from build123d import *

# Parameters (mm, degrees)
SKETCH1_R           = 4
SKETCH1_R_2         = 2.525
BOSS_EXTRUDE1_DEPTH = 5.1
BOSS_EXTRUDE2_DEPTH = 6.4
SKETCH3_R           = 2.5
BOSS_EXTRUDE5_DEPTH = 1.1


with BuildPart() as part:
    # Sketch1 → Boss-Extrude1 (new body)
    with BuildSketch(Plane.XY):
        Circle(SKETCH1_R)
        Circle(SKETCH1_R_2, mode=Mode.SUBTRACT)
    extrude(amount=BOSS_EXTRUDE1_DEPTH)

    # Sketch2 → Boss-Extrude2 (add)
    with BuildSketch(Plane(origin=(0, 0, 0), x_dir=(-1, 0, 0), z_dir=(0, 0, -1))):
        Polygon((-1.7, 3.4), (-1.7, 1.7), (-3.4, 1.7), (-3.4, -1.7), (-1.7, -1.7), (-1.7, -3.4), (1.7, -3.4), (1.7, -1.7), (3.4, -1.7), (3.4, 1.7), (1.7, 1.7), (1.7, 3.4), align=None)
        with BuildLine():
            Line((-1.05, 2.45), (-1.05, 1.55))
            ThreePointArc((-1.05, 1.55), (-1.196446609, 1.196446609), (-1.55, 1.05))
            Line((-1.55, 1.05), (-2.45, 1.05))
            Line((-2.45, 1.05), (-2.45, -1.05))
            Line((-2.45, -1.05), (-1.55, -1.05))
            ThreePointArc((-1.55, -1.05), (-1.196446609, -1.196446609), (-1.05, -1.55))
            Line((-1.05, -1.55), (-1.05, -2.45))
            Line((-1.05, -2.45), (1.05, -2.45))
            Line((1.05, -2.45), (1.05, -1.55))
            ThreePointArc((1.05, -1.55), (1.196446609, -1.196446609), (1.55, -1.05))
            Line((1.55, -1.05), (2.45, -1.05))
            Line((2.45, -1.05), (2.45, 1.05))
            Line((2.45, 1.05), (1.55, 1.05))
            ThreePointArc((1.55, 1.05), (1.196446609, 1.196446609), (1.05, 1.55))
            Line((1.05, 1.55), (1.05, 2.45))
            Line((1.05, 2.45), (-1.05, 2.45))
        make_face(mode=Mode.SUBTRACT)
    extrude(amount=BOSS_EXTRUDE2_DEPTH)

    # Sketch3 → Boss-Extrude5 (add)
    with BuildSketch(Plane(origin=(0, 0, 0), x_dir=(-1, 0, 0), z_dir=(0, 0, -1))):
        Circle(SKETCH3_R)
        Polygon((-0.80736121, 2.151247078), (-0.80736121, 0.83443077), (-2.19666282, 0.83443077), (-2.19666282, -0.796488511), (-0.80736121, -0.796488511), (-0.80736121, -2.18579012), (0.78731542, -2.18579012), (0.78731542, -0.796488511), (2.152455262, -0.796488511), (2.152455262, 0.83443077), (0.78731542, 0.83443077), (0.78731542, 2.151247078), align=None, mode=Mode.SUBTRACT)
    extrude(amount=-BOSS_EXTRUDE5_DEPTH)


solid = part.part
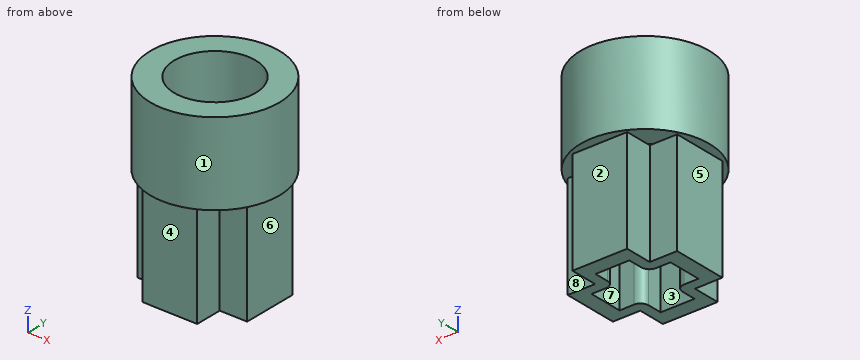
Source: CAD feature listing. Evaluate the final solid. Frame: model axes, mm. Face numbers are marked on the shaded views. A direction names the side the tool comes from. Round coordinates to 2 decimals unless told otherwise and drop trailing zeros. Loops run counter-clockwise (first coordinate to the right, second up) from the corner with the lowest first, then second, coordinate; pieces in that order, holes last. Notation, with made-up numbers: M -13.5,-25.75 L 10.5,-25.75 A17 cw 10.5,-5.75 Z; hole C 6.5,14.5 d5. An arc over 180 degrees is marked long. Return JSON: item names as keys, results as strings. Group by question number.
1. Pin query (flat end, axial travel): pin 1 (1.2 mm diameter, centred on x = 1.5, z = 1, fed in from -Y); pin 2 (2.5 mm diameter, centred on x = 1, y = -1, fed in from -Z); pin 3 (2 mm diameter, centred on y = 0, z = -3, fed in from +X); pin 4 (0.5 mm diameter, centred on x = -1, y = 2, fed in from +Z). Return the tip coordinate at first contact, or that it passes through.
2. Mould query, pull axis X, two halves, no side actions, for the marked faces 1, 2 and 3. Classes: released by +X, released by -X, zero draft, split by the parting line, or undercut.
3. Section query A-A on y = 0. Output: boundary loops of the cut face in (x, z) (3 decimals), and give its area (3 significant figures).
4. Section query C-C on z = -2.75. Output: boundary loops of the cut face in (x, y), and give its area (3 significant figures).
5. Section query D-D on y = -3.25. Output: boundary loops of the cut face in (x, z), and give its area (3 significant figures).
6. Section query B-B on x = 0. Output: boundary loops of the cut face in (y, z) (3 decimals).
7. Material intervals for line 1 along X through (y, z) = (-1.75, -4.75); line 2 along Y through (x, z) = (0, 4.05) (3 decimals); line 3 along Y through (x, z) = (-1, -3.25), sorted ascending. Write a range as from..to.
8. Reachability of the marked faces 4, 5, 6, 7 and 8 from +Z, -Z, +X, -X, +Y, -Y: full face, straight path, thin tool, end or side. Return the list, or none.
Checks:
{
 "1": {"pin 1": "stops at y = -3.9", "pin 2": "stops at z = -6.4", "pin 3": "stops at x = 3.4", "pin 4": "stops at z = 1.1"},
 "2": {"face 1": "split by the parting line", "face 2": "zero draft", "face 3": "undercut"},
 "3": {"outline": "M -4,0 L -3.4,0 L -3.4,-6.4 L -2.45,-6.4 L -2.45,0 L -2.152,0 L -2.152,1.1 L -2.5,1.1 L -2.5,0 L -2.525,0 L -2.525,5.1 L -4,5.1 Z; M 2.197,0 L 2.45,0 L 2.45,-6.4 L 3.4,-6.4 L 3.4,0 L 4,0 L 4,5.1 L 2.525,5.1 L 2.525,0 L 2.5,0 L 2.5,1.1 L 2.197,1.1 Z", "area": "27.9 mm²"},
 "4": {"outline": "M -3.4,-1.7 L -1.7,-1.7 L -1.7,-3.4 L 1.7,-3.4 L 1.7,-1.7 L 3.4,-1.7 L 3.4,1.7 L 1.7,1.7 L 1.7,3.4 L -1.7,3.4 L -1.7,1.7 L -3.4,1.7 Z; hole M -2.45,-1.05 L -1.55,-1.05 A0.5 cw -1.05,-1.55 L -1.05,-2.45 L 1.05,-2.45 L 1.05,-1.55 A0.5 cw 1.55,-1.05 L 2.45,-1.05 L 2.45,1.05 L 1.55,1.05 A0.5 cw 1.05,1.55 L 1.05,2.45 L -1.05,2.45 L -1.05,1.55 A0.5 cw -1.55,1.05 L -2.45,1.05 Z", "area": "18.3 mm²"},
 "5": {"outline": "M -2.33,0 L -1.7,0 L -1.7,-6.4 L 1.7,-6.4 L 1.7,0 L 2.33,0 L 2.33,5.1 L -2.33,5.1 Z", "area": "45.5 mm²"},
 "6": {"outline": "M -4,0 L -3.4,0 L -3.4,-6.4 L -2.45,-6.4 L -2.45,0 L -2.186,0 L -2.186,1.1 L -2.5,1.1 L -2.5,0 L -2.525,0 L -2.525,5.1 L -4,5.1 Z; M 2.151,0 L 2.45,0 L 2.45,-6.4 L 3.4,-6.4 L 3.4,0 L 4,0 L 4,5.1 L 2.525,5.1 L 2.525,0 L 2.5,0 L 2.5,1.1 L 2.151,1.1 Z"},
 "7": {"line 1": "x = -1.7..-1.05, 1.05..1.7", "line 2": "y = -4..-2.525, 2.525..4", "line 3": "y = -3.4..-2.45, 2.45..3.4"},
 "8": {"face 4": "-Z, +X, -X, -Y", "face 5": "-Z, -X, +Y, -Y", "face 6": "-Z, +X, +Y, -Y", "face 7": "-Z", "face 8": "-Z, +X, +Y"}
}
